Read the model definition and answer for the solid it produces. Units are mm, in the model's axes. Face numbers are marked on the shaded views. Give positions to 0.01 mm unless a question says otherwise; leave off trailing zeros. Loops run counter-clockwise (first coordinate to the right, second up) from the corner with the lowest first, then second, coordinate; pieces in that order, holes last.
(1) Straight lines are drawn through the part: probe 1 along X at (y, z) = (71.5, 0.6); probe 2 along X at (y, z) = (0, 1.75); probe 3 along Y at (x, z) = (5, 4.25). For each, find the intervals that lie inside material, in ascending order.
(2) Find section B-B, the plane x = 0. Write down the section's boundary in (y, z), then the cut area to 3 significant figures.
(3) Each of these flat-tipped pins is pushed along its axis until it touches: P1, Ø1, axis at y = 15.5, z = 2, coming from the +X side; P2, Ø1.6, axis at y = 10.5, z = 2, coming from the -X side; P3, Ø8, axis at x = -12, y = 70, coming from the +Z side; P4, Ø2, axis at y = 63.5, z = 0.5, coming from the -X side. Where does it stop, or does it pass through?
(4) Find section A-A, the plane z = 1.8. Write down the section's boundary in (x, y).
(5) Determine the mould class of the marked faces 1, 2 and 3 for opening direction Y: pulls with the +Y half, pulls with the -Y half, needs draft (parallel to the pull), parting line crosses it, or undercut.
Solid Edge part; units mm, degrees
sketch "Sketch1" plane through (0, 0, 0) normal (0, 0, 1) x (1, 0, 0)
  circle A0 centre (12, 70) radius 3
  arc A1 (0, -17) -> (17, 0) centre (0, 0) ccw
  arc A2 (17, 0) -> (17.9976, 69.8286) centre (2461.5, 0) cw
  arc A3 (12, 76) -> (17.9976, 69.8286) centre (12, 70) cw
  line L0 (12, 76) -> (0, 76)
  line L1 (0, 10) -> (0, 76)
  arc A4 (0, 10) -> (0, -10) centre (0, 0) cw
  line L2 (0, -17) -> (0, -10)
  dimension "D1" = 12
extrude "Protrusion1" add sketch "Sketch1" along normal blind 5
mirror "Mirror1" about plane through (0, 0, 0) normal (1, 0, 0) of "Protrusion1"
sketch "Sketch2" plane through (0, 14.5, 5) normal (0, 0, 1) x (1, 0, 0)
  arc A0 (-2, -4.702) -> (2, -4.702) centre (0, -14.5) cw
  line L0 (2, -2.702) -> (2, -4.702)
  line L1 (-2, -2.702) -> (2, -2.702)
  line L2 (-2, -4.702) -> (-2, -2.702)
  dimension "D1" = 2
  dimension "D2" = 2
extrude "ExtrudedCutout_1" cut sketch "Sketch2" against normal blind 9.3641
fillet "Round_1" radius 0.2 12 edges at (17.2494, 34.9179, 0) (16.3028, 74.1816, 0) (0, 76, 0) (-16.3028, 74.1816, 0) (-17.2494, 34.9179, 0) (0, -17, 0) (17.2494, 34.9179, 5) (16.3028, 74.1816, 5) (0, 76, 5) (-16.3028, 74.1816, 5) (-17.2494, 34.9179, 5) (0, -17, 5)
properties material "Steel"
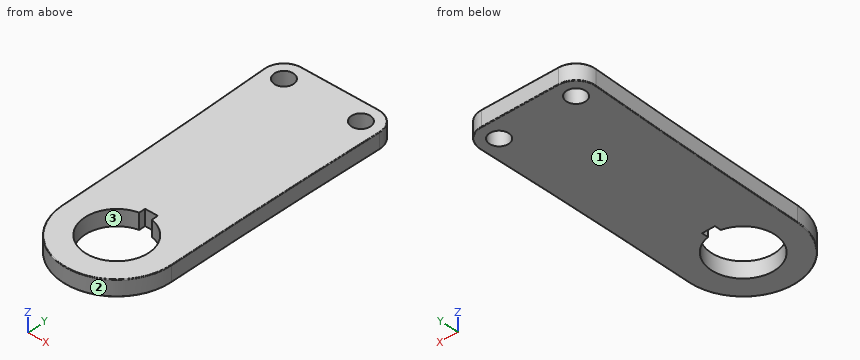
Entries:
1. probe 1: x = -17.81 to -14.6, -9.4 to 9.4, 14.6 to 17.81
1. probe 2: x = -17 to -10, 10 to 17
1. probe 3: y = -16.25 to -8.66, 8.66 to 76
2. outline: (-17, 0.2) arc R0.2 ccw to (-16.8, 0) - (-10, 0) - (-10, 5) - (-16.8, 5) arc R0.2 ccw to (-17, 4.8) - close; (11.8, 0) - (75.8, 0) arc R0.2 ccw to (76, 0.2) - (76, 4.8) arc R0.2 ccw to (75.8, 5) - (11.8, 5) - close
2. area: 356 mm2
3. P1: stops at x = 17.05
3. P2: stops at x = -17.03
3. P3: stops at z = 5
3. P4: stops at x = -17.85
4. outline: (-18, 69.83) arc R2444.5 cw to (-17, 0) arc R17 ccw to (17, 0) arc R2444.5 cw to (18, 69.83) arc R6 ccw to (12, 76) - (-12, 76) arc R6 ccw to start; hole circle Ø6 at (-12, 70); hole (-2, 9.8) arc R10 ccw (long way) to (2, 9.8) - (2, 11.8) - (-2, 11.8) - close; hole circle Ø6 at (12, 70)
5. face 1: needs draft
5. face 2: pulls with the -Y half
5. face 3: undercut
